Geometry: final body of the model. Coordinates: model frame, mm. Give positions to 0.01 mm unless a question says otherwise; leave off trailing zeros. Loops run counter-clockwise (first coordinate to the right, second up) from the corner with the lowest first, then second, coordinate; pieces in that order, holes last. Notation, with made-up numbers: (79, 69) -> (83, 69) arc R12 ccw to (83, 92) -> close; hole circle Ø4 at (47.25, 67). An arc over 180 degrees is marked (long way). One line per question, with ' | ' between items. Start each with the question number.
Item 1: Section A-A on z = 2.75. Return loops of the section in (x, y), then the cut area to 3 significant figures.
Item 2: Material intervals for line 1 along Y through (x, z) = (0, 2.25); line 2 along Y through (x, z) = (-3.75, 2.5); line 3 along X through (y, z) = (-2.5, -0.25), sorted ascending. Write a range as [from, to].
Item 3: Pin query (flat end, axial travel): P1, Ø3, axis at y = 2, z = 1, coming from the -X side. Return the tip coordinate at first contact, or that it passes through.
from build123d import *

# Parameters (mm, degrees)
SKETCH1_R           = 4.5
BOSS_EXTRUDE3_DEPTH = 4.5
SKETCH3_OUTSIDE_W   = 43.092
SKETCH3_OUTSIDE_H   = 40.68
SKETCH3_OUTSIDE_R   = 7.794228634
CUT_EXTRUDE5_DEPTH  = 9
CUT_EXTRUDE5_TAPER  = 45


with BuildPart() as part:
    # Sketch1 → Boss-Extrude3 (new body, symmetric)
    with BuildSketch(Plane.XY):
        Polygon((9, 0), (4.5, 7.794228634), (-4.5, 7.794228634), (-9, 0), (-4.5, -7.794228634), (4.5, -7.794228634), align=None)
        Circle(SKETCH1_R, mode=Mode.SUBTRACT)
    extrude(amount=BOSS_EXTRUDE3_DEPTH, both=True)

    # Sketch3 outside → Cut-Extrude5 (cut)
    with BuildSketch(Plane.XY.offset(4.5)):
        Rectangle(SKETCH3_OUTSIDE_W, SKETCH3_OUTSIDE_H)
        Circle(SKETCH3_OUTSIDE_R, mode=Mode.SUBTRACT)
    cut_extrude5 = extrude(amount=-CUT_EXTRUDE5_DEPTH, taper=CUT_EXTRUDE5_TAPER, mode=Mode.SUBTRACT)

    # Mirror2: Cut-Extrude5 across plane
    add(cut_extrude5.mirror(Plane.XY), mode=Mode.SUBTRACT)


solid = part.part
Result sheet:
1) outline: (-9, 0) -> (-4.5, -7.79) -> (4.5, -7.79) -> (9, 0) -> (4.5, 7.79) -> (-4.5, 7.79) -> close; hole circle Ø9 at (0, 0) | area: 147 mm²
2) line 1: y = [-7.79, -4.5], [4.5, 7.79] | line 2: y = [-7.79, -2.49], [2.49, 7.79] | line 3: x = [-7.56, -3.74], [3.74, 7.56]
3) P1: stops at x = -8.71
